Read the model definition and answer for the solid it produces. Units are mm, in the model's axes. A direction names the side the tool comes from. Coordinates: 2 decimals unless noted, no trailing zeros. Loops run counter-clockwise (first coordinate to the right, second up) from the corner with the lowest first, then second, coordinate; pieces in that order, holes last. Notation, with made-up numbers: M 70.25,-17 L 74.25,-17 A13 ccw 74.25,-13 Z; hole C -24,28.5 d10. An arc over 180 degrees is marked long. Put each result on its own line as item: value.
from build123d import *

# Parameters (mm, degrees)
F0_W     = 50.8
F0_H     = 177.8
F1_DEPTH = 3.175
F3_DEPTH = 76.2
F5_DEPTH = 3.175
F7_D     = 6.7564
F7_DEPTH = 29.21
F7_TIP   = 2.0298273432


with BuildPart() as f1:
    # F0 (on Top) → F1 (new body)
    with BuildSketch(Plane.XY):
        Polygon((0, 228.6), (0, 177.8), (50.8, 177.8), (177.8, 177.8), (177.8, 228.6), align=None)
        with Locations((25.4, 88.9)):
            Rectangle(F0_W, F0_H)
    extrude(amount=F1_DEPTH)

    # F2 (on face) → F3 (join)
    with BuildSketch(Plane.XY.offset(3.175)):
        Polygon((3.175, 0), (3.175, 225.425), (177.8, 225.425), (177.8, 228.6), (0, 228.6), (0, 0), align=None)
    extrude(amount=F3_DEPTH)

    # F4 (on face) → F5 (join)
    with BuildSketch(Plane.XY.offset(79.375)):
        Polygon((177.8, 228.6), (0, 228.6), (0, 0), (3.175, 0), (3.175, 225.425), (177.8, 225.425), align=None)
        Polygon((177.8, 177.8), (177.8, 225.425), (3.175, 225.425), (3.175, 0), (50.8, 0), (50.8, 177.8), align=None)
    extrude(amount=F5_DEPTH)

    # F7
    with Locations(Plane.XY.offset(82.55)):
        with Locations((26.9875, 25.4), (26.9875, 50.8), (26.9875, 76.2), (26.9875, 101.6), (26.9875, 127), (26.9875, 152.4), (26.9875, 177.8), (50.8, 201.6125), (76.2, 201.6125), (101.6, 201.6125), (127, 201.6125), (152.4, 201.6125)):
            Hole(F7_D / 2, depth=F7_DEPTH)
            with Locations((0, 0, -(F7_DEPTH + F7_TIP / 2))):  # 118° drill point
                Cone(0, F7_D / 2, F7_TIP, mode=Mode.SUBTRACT)


solid = f1.part
1) Straight lines are drawn through the part: line 1 (Y direction, x = 101.6, z = 81.5); line 2 (Z direction, x = 22.5, y = 70) (3 decimals); line 3 (Y direction, x = 25, z = 37.5) (3 decimals). For each, find the intervals that lie inside material, in ascending order. Write a range as [from, to].
Answer list:
line 1: y = [177.8, 198.23], [204.99, 228.6]
line 2: z = [0, 3.175], [79.375, 82.55]
line 3: y = [225.425, 228.6]
2) Find section C-C, the plane z = 62.5. Write down the section's boundary in (x, y) (3 decimals).
Answer list:
outline: M 0,0 L 3.175,0 L 3.175,225.425 L 177.8,225.425 L 177.8,228.6 L 0,228.6 Z
3) Given pin 1 Ø23 at (x, z) = (88, 44.5) entering from -Y (3 decimals); pin 2 Ø4 at (x, y) = (26.99, 177.8) entering from +Z (3 decimals); pin 3 Ø1.6 at (y, z) = (89, 80.5) entering from +X; pin 4 Ø10 at (x, y) = (59.5, 98.5) entering from +Z, each flat-ended and moving along its own axis, determine where each tip first touches the part or whether it passes through.
Answer list:
pin 1: stops at y = 225.425
pin 2: stops at z = 3.175
pin 3: stops at x = 50.8
pin 4: passes through
4) Find section A-A, the plane y = 152.4. Write down the section's boundary in (x, z) (3 decimals).
Answer list:
outline: M 0,0 L 50.8,0 L 50.8,3.175 L 3.175,3.175 L 3.175,79.375 L 23.609,79.375 L 23.609,82.55 L 0,82.55 Z; M 30.366,79.375 L 50.8,79.375 L 50.8,82.55 L 30.366,82.55 Z
5) Find section D-D, the plane x = 37. Write down the section's boundary in (y, z) (3 decimals).
Answer list:
outline: M 0,0 L 228.6,0 L 228.6,82.55 L 0,82.55 L 0,79.375 L 225.425,79.375 L 225.425,3.175 L 0,3.175 Z
6) Determine the mould class of faces 1 (the flat face through (48, 141, 82.55)), 2 (the flat face through (3.175, 111, 41)), 3 (the flat face through (50, 139, 79.375)), 4 (the cylindrical face through (25.429, 149.403, 80.94)) for opening direction Z: released by +Z, released by -Z, zero draft, split by the parting line, or undercut.
Answer list:
face 1: released by +Z
face 2: undercut
face 3: undercut
face 4: zero draft
7) Which of the six approach directions +Z, -Z, +X, -X, +Y, -Y give full straight-line access (tool end or side, diameter ignored) to faces 5 (the flat face through (90, 228.6, 41)), 6 (the flat face through (50, 139, 3.175)), 7 (the cylindrical face through (25.171, 104.449, 80.94))?
Answer list:
face 5: +Z, -Z, +X, -X, +Y
face 6: +X, -Y
face 7: +Z
8) Find section B-B, the plane x = 127. Write down the section's boundary in (y, z) (3 decimals).
Answer list:
outline: M 177.8,0 L 228.6,0 L 228.6,82.55 L 204.991,82.55 L 204.991,79.375 L 225.425,79.375 L 225.425,3.175 L 177.8,3.175 Z; M 177.8,79.375 L 198.234,79.375 L 198.234,82.55 L 177.8,82.55 Z
